The drawing under review shows one solid part. Ordinate dimensions are in mm from its lowest x, y, z. Coordinates: 2 decimals unless noted, no trailing zeros. Write each loop counter-clockwise with the first axis right and the second up, starting at its lowest first coordinate (ties: lowest second). Pieces come first, ordered by that corner, then holes. Notation, with made-up numbers: (-20.75, -6) -> (20.25, -6) arc R23 cw to (20.25, 21) -> close; hole circle Ø2 at (37.25, -8). An arc over 180 degrees is marked (long way). One line per question, with ' | ' between items. Start each with the question number.
Q1. Wall thickness on probe 1 along Z at (x, y) = (26.5, 22); probe 2 along Z at (x, y) = (118, 3); probe 3 along X at (y, z) = (19.5, 90): over which ranges is each line inside the solid? List them lowest first.
Q2. Add section A-A on y = 2. State the section outline as (x, z) points.
Q3. Add section C-C on x = 43.5. State the section outline as (y, z) points, and give its area (3 significant figures).
Q4. Add section B-B on z = 65. State the section outline as (x, y) points.
Q5. For P1, Ø2, axis at y = 7.5, z = 69.5, coming from the +X side; P2, Ø2, axis at x = 51, y = 7.5, coming from the +Z side; P3, Ø5, axis at x = 32.5, y = 16, coming from the +Z side, all flat-tipped, find the tip position at first contact; note any pin that passes through.
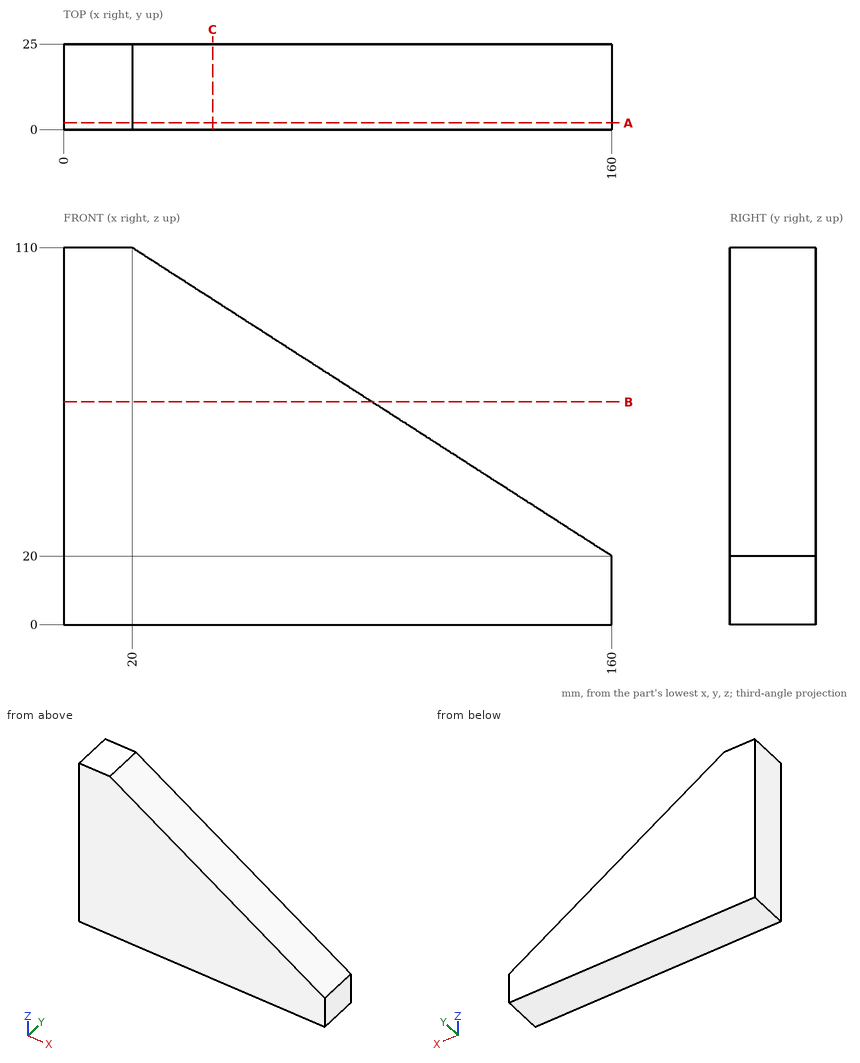
Output values:
1) probe 1: z = 0 to 105.82 | probe 2: z = 0 to 47 | probe 3: x = 0 to 51.11
2) outline: (0, 0) -> (160, 0) -> (160, 20) -> (20, 110) -> (0, 110) -> close
3) outline: (0, 0) -> (25, 0) -> (25, 94.89) -> (0, 94.89) -> close | area: 2,370 mm2
4) outline: (0, 0) -> (90, 0) -> (90, 25) -> (0, 25) -> close
5) P1: stops at x = 84.56 | P2: stops at z = 90.71 | P3: stops at z = 103.57
